Could you check a few things on this model? Use its own coordinates, in mm. Round coordinates to 2 decimals unless told otherwise and drop trailing zeros. Write each loop counter-clockwise with the first axis right and the second up, starting at its lowest first coordinate (ties: lowest second). Pieces come first, ordered by that corner, then holes. Notation, with made-up numbers: (42.5, 1) -> (81.5, 1) arc R13 cw to (81.5, 5) -> close; hole circle Ø10 at (44, -7.5). An arc over 180 degrees is marked (long way). Return JSON: item names as keys, results as strings.
Autodesk Inventor part; units mm, degrees
ref_plane "YZ Plane" through (0, 0, 0) normal (1, 0, 0) x (0, 1, 0)
ref_plane "XZ Plane" through (0, 0, 0) normal (0, 1, 0) x (-1, 0, 0)
ref_plane "XY Plane" through (0, 0, 0) normal (0, 0, 1) x (1, 0, 0)
sketch "Esboço1" plane through (0, 0, 0) normal (1, 0, 0) x (0, 1, 0)
  line L0 (1012, 0) -> (1012, -72)
  line L1 (0, -72) -> (0, 0)
  line L2 (1012, 0) -> (946, 0)
  line L3 (946, 0) -> (946, 6)
  line L4 (946, 6) -> (886, 6)
  line L5 (886, 6) -> (886, 0)
  line L6 (0, 0) -> (66, 0)
  line L7 (66, 0) -> (66, 6)
  line L8 (66, 6) -> (126, 6)
  line L9 (126, 6) -> (126, 0)
  line L10 (126, 0) -> (886, 0)
  line L11 (1012, -72) -> (946, -72)
  line L12 (946, -72) -> (946, -78)
  line L13 (946, -78) -> (886, -78)
  line L14 (886, -78) -> (886, -72)
  line L15 (886, -72) -> (126, -72)
  line L16 (126, -72) -> (126, -78)
  line L17 (126, -78) -> (66, -78)
  line L18 (66, -78) -> (66, -72)
  line L19 (66, -72) -> (0, -72)
  dimension "d1" = 72
  dimension "d2" = 66
  dimension "d3" = 6
  dimension "d4" = 60
  dimension "d7" = 6
  dimension "d8" = 6
  dimension "d9" = 60
  dimension "d10" = 66
  dimension "d11" = 6
  dimension "d12" = 66
  dimension "d13" = 6
  dimension "d14" = 60
  dimension "d17" = 1012
extrude "Extrusão1" add sketch "Esboço1" along normal blind 4
sketch "Esboço2" plane through (4, 0, 0) normal (1, 0, 0) x (0, 0, -1)
  point P0 (0, 0)
properties part number "FUNDO CONTRA"
1) I want a section at A-A, the plane x = 2.65. Please give me the cut outline in (y, z), and give its area (3 significant figures).
Return value:
{"outline": "(0, -72) -> (66, -72) -> (66, -78) -> (126, -78) -> (126, -72) -> (886, -72) -> (886, -78) -> (946, -78) -> (946, -72) -> (1012, -72) -> (1012, 0) -> (946, 0) -> (946, 6) -> (886, 6) -> (886, 0) -> (126, 0) -> (126, 6) -> (66, 6) -> (66, 0) -> (0, 0) -> close", "area": "74,300 mm²"}
2) I want a section at B-B, the plane y = 840. Please give me the cut outline in (x, z), and give its area (3 significant figures).
Return value:
{"outline": "(0, -72) -> (4, -72) -> (4, 0) -> (0, 0) -> close", "area": "288 mm²"}
3) Will these pins go through, and if not, where does the flat tip stop? pin 1 Ø2 at (x, y) = (1.5, 526) entering from -Z; pin 2 Ø2 at (x, y) = (2, 17.5) entering from +Z; pin 3 Ø2 at (x, z) = (2, -74) entering from -Y.
Return value:
{"pin 1": "z = -72", "pin 2": "z = 0", "pin 3": "y = 66"}
4) If I drill on probe 1 along Y at (x, z) = (0.45, 2); probe 2 along Z at (x, y) = (3.35, 534), over which ranges is the centre line in solid material (lowest first)? Write a range as [from, to].
Return value:
{"probe 1": "[66, 126], [886, 946]", "probe 2": "[-72, 0]"}
